from build123d import *

# Parameters (mm, degrees)
SKETCH1_W               = 120
SKETCH1_H               = 100
BOSS_EXTRUDE1_DEPTH     = 100
SKETCH2_W               = 60
SKETCH2_H               = 70
CUT_EXTRUDE2_DEPTH      = 101
CUT_EXTRUDE2_DEPTH_BACK = 1
SKETCH3_R               = 4
CUT_EXTRUDE3_DEPTH      = 51
CUT_EXTRUDE3_DEPTH_BACK = 51
SKETCH5_R               = 4
CUT_EXTRUDE4_DEPTH      = 61
CUT_EXTRUDE4_DEPTH_BACK = 61
SKETCH6_R               = 6
CUT_EXTRUDE5_DEPTH      = 61
CUT_EXTRUDE5_DEPTH_BACK = 61
CUT_EXTRUDE7_START      = -20
SKETCH7_R               = 7
CUT_EXTRUDE7_DEPTH      = 10


with BuildPart() as part:
    # Sketch1 → Boss-Extrude1 (new body)
    with BuildSketch(Plane.XY):
        Rectangle(SKETCH1_W, SKETCH1_H)
    extrude(amount=BOSS_EXTRUDE1_DEPTH)

    # Sketch2 → Cut-Extrude2 (cut, two sides)
    with BuildSketch(Plane.XY) as cut_extrude2_sk:
        Polygon((-60, -20), (-40, -50), (-60, -50), align=None)
        with Locations((0, 15)):
            Rectangle(SKETCH2_W, SKETCH2_H)
        Polygon((60, -50), (40, -50), (60, -20), align=None)
    extrude(amount=CUT_EXTRUDE2_DEPTH, mode=Mode.SUBTRACT)
    extrude(cut_extrude2_sk.sketch, amount=-CUT_EXTRUDE2_DEPTH_BACK, mode=Mode.SUBTRACT)

    # Sketch3 → Cut-Extrude3 (cut, two sides)
    with BuildSketch(Plane(origin=(0, 0, 0), x_dir=(1, 0, 0), z_dir=(0, 1, 0))) as cut_extrude3_sk:
        with Locations((0, -85)):
            Circle(SKETCH3_R)
        with Locations((0, -15)):
            Circle(SKETCH3_R)
    extrude(amount=CUT_EXTRUDE3_DEPTH, mode=Mode.SUBTRACT)
    extrude(cut_extrude3_sk.sketch, amount=-CUT_EXTRUDE3_DEPTH_BACK, mode=Mode.SUBTRACT)

    # Sketch5 → Cut-Extrude4 (cut, two sides)
    with BuildSketch(Plane(origin=(0, 0, 0), x_dir=(0, 0, -1), z_dir=(1, 0, 0))) as cut_extrude4_sk:
        with Locations((-91, 15)):
            Circle(SKETCH5_R)
        with Locations((-9, 15)):
            Circle(SKETCH5_R)
    extrude(amount=CUT_EXTRUDE4_DEPTH, mode=Mode.SUBTRACT)
    extrude(cut_extrude4_sk.sketch, amount=-CUT_EXTRUDE4_DEPTH_BACK, mode=Mode.SUBTRACT)

    # Sketch6 → Cut-Extrude5 (cut, two sides)
    with BuildSketch(Plane(origin=(0, 0, 0), x_dir=(0, 0, -1), z_dir=(1, 0, 0))) as cut_extrude5_sk:
        with Locations((-50, 15)):
            Circle(SKETCH6_R)
    extrude(amount=CUT_EXTRUDE5_DEPTH, mode=Mode.SUBTRACT)
    extrude(cut_extrude5_sk.sketch, amount=-CUT_EXTRUDE5_DEPTH_BACK, mode=Mode.SUBTRACT)

    # Sketch7 → Cut-Extrude7 (cut)
    with BuildSketch(Plane(origin=(0, 0, 0), x_dir=(1, 0, 0), z_dir=(0, 1, 0)).offset(CUT_EXTRUDE7_START)):
        with Locations((0, -85)):
            Circle(SKETCH7_R)
        with Locations((0, -15)):
            Circle(SKETCH7_R)
    extrude(amount=-CUT_EXTRUDE7_DEPTH, mode=Mode.SUBTRACT)


solid = part.part
Can you work these out from the model? Positions are in its coordinate system, mm. A direction names the side the tool comes from. Give positions to 0.01 mm unless a question says otherwise; leave off trailing zeros. Loops run counter-clockwise (first coordinate to the right, second up) from the corner with the lowest first, then second, coordinate; pieces in that order, holes last. Notation, with made-up numbers: (40.5, 65.25) -> (56.5, 65.25) arc R32 cw to (56.5, 96.25) -> close; hole circle Ø11 at (-10, 66). An arc over 180 degrees is marked (long way). Write item = value, one per line.
1) Will these pins go through, and if not, where does the flat tip stop? pin 1 (5 mm diameter, centred on y = 15, z = 9, fed in from +X); pin 2 (4 mm diameter, centred on x = 1.5, z = 82, fed in from +Y); pin 3 (15.5 mm diameter, centred on x = -1.5, z = 16, fed in from +Y).
Check result:
pin_1 = through
pin_2 = -30
pin_3 = -20
2) Suppose I cut it at C-C on z = 50. Write out the boundary of the cut face in (x, y).
Check result:
outline = (-60, -20) -> (-40, -50) -> (40, -50) -> (60, -20) -> (60, 9) -> (30, 9) -> (30, -20) -> (-30, -20) -> (-30, 9) -> (-60, 9) -> close; (-60, 21) -> (-30, 21) -> (-30, 50) -> (-60, 50) -> close; (30, 21) -> (60, 21) -> (60, 50) -> (30, 50) -> close
3) I need wall thicknesses on L1, parallel to Z at x = 0, y = -26.25; L2, parallel to Z at x = 52.75, y = 15; L3, parallel to X at y = 40, z = 54.5. Which ranges of each line are inside material? Lowest first, please. Write a range as from..to.
Check result:
L1 = 0..8, 22..78, 92..100
L2 = 0..5, 13..44, 56..87, 95..100
L3 = -60..-30, 30..60
4) Suppose I cut it at D-D on x = 34. Write out the boundary of the cut face in (y, z).
Check result:
outline = (-50, 0) -> (50, 0) -> (50, 100) -> (-50, 100) -> close; hole circle Ø12 at (15, 50); hole circle Ø8 at (15, 9); hole circle Ø8 at (15, 91)
5) For faces 4 (the cylindrical face through (-0.91, -24.93, 78.06)), 5 (the flat face through (-30, 7, 49)), 6 (the flat face through (45, 50, 49)), which set-ups out of +Z, -Z, +X, -X, +Y, -Y let a thin tool reach every point of the face, with its end or its side?
Check result:
face_4 = +Y
face_5 = +Z, -Z, +Y
face_6 = +Z, -Z, +X, -X, +Y
6) Suppose I cut it at A-A on y = -3. Write out the boundary of the cut face in (x, z), then the cut area to 3 significant figures.
Check result:
outline = (-60, 0) -> (-30, 0) -> (-30, 100) -> (-60, 100) -> close; (30, 0) -> (60, 0) -> (60, 100) -> (30, 100) -> close
area = 6,000 mm2
7) Thinking about a two-plate mould opening in Z: for faces 1 (the flat face through (-1, -22, 0)), 2 (the flat face through (3, -30, 18)), 3 (the flat face through (0, -20, 49)), which applies, released by +Z, released by -Z, zero draft, split by the parting line, or undercut?
Check result:
face_1 = released by -Z
face_2 = undercut
face_3 = zero draft
8) Suppose I cut it at B-B on x = 0. Write out the boundary of the cut face in (y, z), then the cut area to 3 significant figures.
Check result:
outline = (-50, 0) -> (-20, 0) -> (-20, 8) -> (-30, 8) -> (-30, 11) -> (-50, 11) -> close; (-50, 19) -> (-30, 19) -> (-30, 22) -> (-20, 22) -> (-20, 78) -> (-30, 78) -> (-30, 81) -> (-50, 81) -> close; (-50, 89) -> (-30, 89) -> (-30, 92) -> (-20, 92) -> (-20, 100) -> (-50, 100) -> close
area = 2,400 mm2
